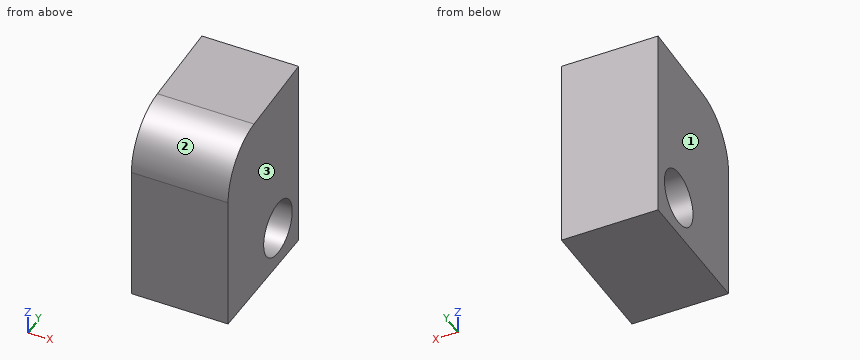
```python
from build123d import *

# Parameters (mm, degrees)
F1_DEPTH = 25.4
F2_R     = 7.311466
F3_DEPTH = 25.4


with BuildPart() as f1:
    # F0 (on Right) → F1 (new body)
    with BuildSketch(Plane.YZ):
        with BuildLine():
            ThreePointArc((-42.888714, 42.924615), (-52.333318, 38.490461), (-56.177065, 28.790571))
            Line((-56.177065, 28.790571), (-56.177065, -7.006547))
            Line((-56.177065, -7.006547), (-20.125262, -7.006547))
            Line((-20.125262, -7.006547), (-20.125262, 44.329979))
            Line((-20.125262, 44.329979), (-42.888714, 42.924615))
        make_face()
    extrude(amount=-F1_DEPTH)

    # F2 (on Right) → F3 (cut)
    with BuildSketch(Plane.YZ):
        with Locations((-30.67892, 3.780983)):
            Circle(F2_R)
    extrude(amount=-F3_DEPTH, mode=Mode.SUBTRACT)


solid = f1.part
```
Could you check a few things on this model? Use its own coordinates, in mm. Face numbers are marked on the shaded views. Give positions to 0.01 mm unless a question says otherwise; leave off trailing zeros. Write each loop counter-clockwise with the first axis right and the second up, starting at its lowest first coordinate (ties: lowest second). Pieces come first, ordered by that corner, then holes. Notation, with made-up numbers: (61, -21.75) - (116, -21.75) arc R8 ccw to (116, -14.75) - close; hole circle Ø8 at (88, 46). An arc over 180 degrees is marked (long way). One line per item, written item: value. Start each with the question number.
Item 1: Imagine slicing it at B-B, the plane z = 10. List the corners of the cut face in (x, y) for me, and give its area (3 significant figures).
Item 2: Please list where these lines run through material, in increasing order: line 1 (Y direction, x = -13.25, z = 3); line 2 (Y direction, x = -9.75, z = 10); line 3 (Z direction, x = -10, y = -25.5). Write a range as from..to.
Item 3: If we mould it in two halves opening along X, with no side actions, what happens to the marked faces 1, 2 and 3? For each: +X half, -X half, draft (parallel to the pull), parting line (faces both ways), or undercut.
Item 4: Imagine slicing it at D-D, the plane y = -49.5. List the corners of the cut face in (x, z) for me.
Item 5: I'm going to push flat-ended pins straight in: pin 1 (5 mm diameter, centred on x = -8.5, y = -49.5, fed in from +Z); pin 2 (4 mm diameter, centred on x = -22.5, z = 37, fed in from -Y). Where does each tip first touch, or does it pass through?
Item 6: Imagine slicing it at C-C, the plane x = -15.75. List the corners of the cut face in (y, z) for me.
Item 7: Imagine slicing it at A-A, the plane y = -31. List the corners of the cut face in (x, z) for me.
Geometry says:
1. outline: (-25.4, -56.18) - (0, -56.18) - (0, -34.52) - (-25.4, -34.52) - close; (-25.4, -26.83) - (0, -26.83) - (0, -20.13) - (-25.4, -20.13) - close
1. area: 720 mm^2
2. line 1: -56.18..-37.95, -23.41..-20.13
2. line 2: -56.18..-34.52, -26.83..-20.13
2. line 3: -7.01..-1.38, 8.94..44
3. face 1: -X half
3. face 2: draft
3. face 3: +X half
4. outline: (-25.4, -7.01) - (0, -7.01) - (0, 40.81) - (-25.4, 40.81) - close
5. pin 1: z = 42.05
5. pin 2: y = -54.74
6. outline: (-56.18, -7.01) - (-20.13, -7.01) - (-20.13, 44.33) - (-42.89, 42.92) arc R14.16 ccw to (-56.18, 28.79) - close; hole circle Ø14.62 at (-30.68, 3.78)
7. outline: (-25.4, -7.01) - (0, -7.01) - (0, -3.52) - (-25.4, -3.52) - close; (-25.4, 11.09) - (0, 11.09) - (0, 43.66) - (-25.4, 43.66) - close
